Read the model definition and answer for the solid it produces. Units are mm, in the model's axes. Coordinates: 2 decimals unless noted, no trailing zeros. Write each loop counter-clockwise with the first axis right and the second up, starting at its lowest first coordinate (ties: lowest second). Pieces come first, ordered by that corner, then holes. Notation, with made-up numbers: (56, -17.5) -> (79, -17.5) arc R15 ccw to (79, -8.5) -> close; hole circle Ø3 at (15, 10.25). An arc over 180 degrees is marked (long way). One line per item, written item: value. Start each with the question number.
1. Consider line 1 along X through (y, z) = (-14.25, -25); line 2 along X through (y, z) = (-11.5, -10); line 3 along Z through (x, y) = (54, -1). Determine where each line is inside the solid, lowest interval first.
2. Find section A-A, the plane y = -17.5. Write down the section's boundary in (x, z), and give its area (3 significant figures).
3. Find section B-B, the plane z = -33.5. Write down the section's boundary in (x, y), and give its area (3 significant figures).
4. Given P1, Ø8, axis at x = 13.5, y = -7, coming from the +Z side; P2, Ø2, axis at y = -19, z = -23.5, coming from the +X side, each flat-ended and moving along its own axis, determine where each tip first touches the part or whether it passes through.
5. Find section C-C, the plane x = 43.5. Write down the section's boundary in (y, z).
6. Find section D-D, the plane y = -3. Write down the section's boundary in (x, z).
```python
from build123d import *

# Parameters (mm, degrees)
F0_W     = 70.552204
F0_H     = 66.001866
F1_DEPTH = 25.4
F2_R     = 25.4
F3_SIZE  = 5.08


with BuildPart() as f1:
    # F0 (on Front) → F1 (new body)
    with BuildSketch(Plane.XZ):
        with Locations((35.276102, -33.000933)):
            Rectangle(F0_W, F0_H)
    extrude(amount=F1_DEPTH)

    # F2
    f2_edges = [f1.edges().sort_by_distance(p)[0] for p in [
        (70.552204, -12.7, 0),
        (0, -12.7, 0),
    ]]
    fillet(f2_edges, radius=F2_R)

    # F3
    f3_edges = [f1.edges().sort_by_distance(p)[0] for p in [
        (70.552204, 0, -45.700933),
        (70.552204, -12.7, -25.4),
        (70.552204, -12.7, -66.001866),
        (70.552204, -25.4, -45.700933),
    ]]
    chamfer(f3_edges, length=F3_SIZE)


solid = f1.part
```
Answer block:
1. line 1: x = 0 to 70.55
1. line 2: x = 5.2 to 65.35
1. line 3: z = -66 to -6
2. outline: (0, -66) -> (65.47, -66) -> (70.55, -60.92) -> (70.55, -25.4) arc R25.4 ccw to (45.15, 0) -> (25.4, 0) arc R25.4 ccw to (0, -25.4) -> close
2. area: 4,370 mm2
3. outline: (0, -20.32) -> (5.08, -25.4) -> (65.47, -25.4) -> (70.55, -20.32) -> (70.55, -5.08) -> (65.47, 0) -> (5.08, 0) -> (0, -5.08) -> close
3. area: 1,740 mm2
4. P1: stops at z = -1.26
4. P2: stops at x = 70.54
5. outline: (-25.4, -66) -> (0, -66) -> (0, -5.08) -> (-5.08, 0) -> (-20.32, 0) -> (-25.4, -5.08) -> close
6. outline: (2.08, -66) -> (65.47, -66) -> (68.47, -63) -> (68.47, -25.4) arc R23.32 ccw to (45.15, -2.08) -> (25.4, -2.08) arc R23.32 ccw to (2.08, -25.4) -> close
